Read the model definition and answer for the solid it produces. Units are mm, in the model's axes. Face numbers are marked on the shaded views. A direction names the side the tool comes from. Round coordinates to 2 decimals unless told otherwise and drop trailing zeros. Write each loop counter-clockwise with the first axis right and the second up, starting at its lowest first coordinate (ties: lowest second). Pieces come first, ordered by that corner, then holes.
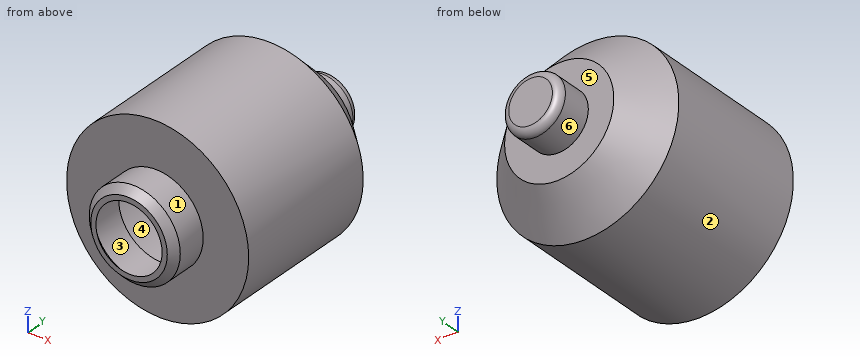
from build123d import *

# Parameters (mm, degrees)
F0_R     = 63.5
F1_DEPTH = 127
F2_R     = 31.75
F3_DEPTH = 25.4
F4_R     = 20.32
F5_DEPTH = 25.4
F6_R     = 5.08
F7_SIZE  = 25.4
F8_SIZE  = 5.08
F9_T     = -2.54


with BuildPart() as f1:
    # F0 (on Front) → F1 (new body)
    with BuildSketch(Plane.XZ):
        with Locations((0, 42.1909095929)):
            Circle(F0_R)
    extrude(amount=F1_DEPTH)

    # F2 (on face) → F3 (join)
    with BuildSketch(Plane.XZ.offset(127)):
        with Locations((0, 42.1909095929)):
            Circle(F2_R)
    extrude(amount=F3_DEPTH)

    # F4 (on face) → F5 (join)
    with BuildSketch(Plane(origin=(0, 0, 0), x_dir=(-1, 0, 0), z_dir=(0, 1, 0))):
        with Locations((0, 42.1909095929)):
            Circle(F4_R)
    extrude(amount=F5_DEPTH)

    # F6
    f6_edges = [f1.edges().sort_by_distance(p)[0] for p in [
        (20.32, 25.4, 42.19091),
    ]]
    fillet(f6_edges, radius=F6_R)

    # F7
    f7_edges = [f1.edges().sort_by_distance(p)[0] for p in [
        (-63.5, 0, 42.19091),
    ]]
    chamfer(f7_edges, length=F7_SIZE)

    # F8
    f8_edges = [f1.edges().sort_by_distance(p)[0] for p in [
        (-31.75, -152.4, 42.19091),
    ]]
    chamfer(f8_edges, length=F8_SIZE)

    # F9
    f9_openings = [f1.faces().sort_by_distance(p)[0] for p in [
        (0, -152.4, 42.19091),
    ]]
    offset(amount=F9_T, openings=f9_openings, kind=Kind.INTERSECTION)


solid = f1.part
Q1. Which of the six approach directions +Z, -Z, +X, -X, +Y, -Y give full straight-line access (tool end or side, diameter ignored) to the marked faces 1 and 2?
Verdict:
face 1: -Y
face 2: +Y, -Y
Q2. Section B-B (y = -116.5) is taken. Determine the outline of the cut face in (x, z).
Verdict:
outline: circle Ø127 at (0, 42.19); hole circle Ø121.92 at (0, 42.19)
Q3. Flat-ended cylindrical pins translate along their axes: pin 1 Ø12 at (y, z) = (-108.5, 44.5) entering from +X; pin 2 Ø3 at (x, z) = (-46, 75) entering from -Y; pin 3 Ø1 at (y, z) = (-104.5, 50) entering from +X; pin 4 Ø4 at (x, y) = (5.5, -45.5) entering from +Z. Find the tip coordinate at first contact, or state that the pin passes through.
Verdict:
pin 1: stops at x = 63.5
pin 2: stops at y = -127
pin 3: stops at x = 63.08
pin 4: stops at z = 105.59
Q4. Straight lines are drawn through the part: probe 1 along Y at (x, z) = (29, 59); probe 2 along Z at (x, y) = (0, 3); probe 3 along Z at (x, y) = (0, -81). For each, find the intervals that lie inside material, in ascending order.
Verdict:
probe 1: y = -127 to -124.46, -2.54 to 0
probe 2: z = 21.87 to 24.41, 59.97 to 62.51
probe 3: z = -21.31 to -18.77, 103.15 to 105.69
Q5. Determine the mould class of the marked faces 3, 4, 5 and 6 for opening direction X: pulls with the +X half, pulls with the -X half, needs draft (parallel to the pull), parting line crosses it, or undercut.
Verdict:
face 3: undercut
face 4: undercut
face 5: needs draft
face 6: parting line crosses it
Q6. Section A-A (y = -11.5) is taken. Determine the outline of the cut face in (x, z).
Verdict:
outline: circle Ø99.2 at (0, 42.19); hole circle Ø92.02 at (0, 42.19)
